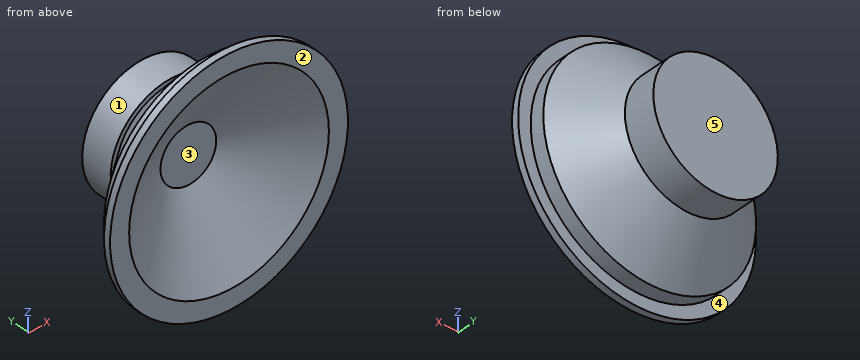
```python
from build123d import *


with BuildPart() as part:
    # Эскиз1 → Повернуть1 (revolve)
    with BuildSketch(Plane(origin=(0, 0, 0), x_dir=(0, 0, -1), z_dir=(1, 0, 0))):
        Polygon((0, 104), (0, 50), (-30, 50), (-107.5, 0), (-128, 0), (-128, 7.5), (-114.5, 7.5), (-114.5, 23), (-62, 69), (-67, 69), (-67, 104), align=None)
    revolve(axis=Axis((0, 0, 0), (0, 1, 0)))


solid = part.part
```
Here's how the part is built. I have some questions about the finished solid (model axes, mm). Face numbers are marked on the shaded views. A direction names the side the tool comes from. Round coordinates to 2 decimals unless told otherwise and drop trailing zeros. Loops run counter-clockwise (first coordinate to the right, second up) from the corner with the lowest first, then second, coordinate; pieces in that order, holes last.
1. Suppose I cut it at A-A, the plane x = 0. Please give me the cut outline in (y, z), and give its area (3 significant figures).
Answers:
outline: (0, -128) - (7.5, -128) - (7.5, -114.5) - (23, -114.5) - (69, -62) - (69, -67) - (104, -67) - (104, 67) - (69, 67) - (69, 62) - (23, 114.5) - (7.5, 114.5) - (7.5, 128) - (0, 128) - (0, 107.5) - (50, 30) - (50, -30) - (0, -107.5) - close
area: 11,400 mm2
2. Thinking about a two-plate mould opening in Z: for the marked faces 1, 2 and 3, which applies, released by +Z, released by -Z, zero draft, split by the parting line, or undercut?
Answers:
face 1: split by the parting line
face 2: zero draft
face 3: undercut
3. If I drill on probe 1 along X at (y, z) = (73.5, -0.5); probe 2 along X at (y, z) = (6, -4); probe 3 along Y at (x, z) = (-59, 26), over which ranges is the centre line in solid material (lowest first)?
Answers:
probe 1: x = -67 to 67
probe 2: x = -127.94 to -98.12, 98.12 to 127.94
probe 3: y = 27.76 to 66.83, 69 to 104
4. Suppose I cut it at B-B, the plane z = 0. Please give me the cut outline in (x, y).
Answers:
outline: (-128, 0) - (-107.5, 0) - (-30, 50) - (30, 50) - (107.5, 0) - (128, 0) - (128, 7.5) - (114.5, 7.5) - (114.5, 23) - (62, 69) - (67, 69) - (67, 104) - (-67, 104) - (-67, 69) - (-62, 69) - (-114.5, 23) - (-114.5, 7.5) - (-128, 7.5) - close
5. For the marked faces 4 and 5, which set-ups out of +Z, -Z, +X, -X, +Y, -Y let a thin tool reach every point of the face, with its end or its side?
Answers:
face 4: +Y
face 5: +Z, -Z, +X, -X, +Y
6. Will these pins go through, and if not, where does the flat tip stop? pin 1 (1.5 mm diameter, centred on x = -60.5, y = 50, fed in from -Z); pin 2 (4 mm diameter, centred on y = 36, z = 8.5, fed in from -X); pin 3 (1 mm diameter, centred on y = 56.5, z = 16, fed in from +X); pin 4 (8 mm diameter, centred on x = 65.5, z = -25, fed in from +Y).
Answers:
pin 1: stops at z = -59.27
pin 2: stops at x = -101.6
pin 3: stops at x = 75.16
pin 4: stops at y = 104
